from build123d import *

# Parameters (mm, degrees)
F0_R     = 4
F1_DEPTH = 2
F2_DEPTH = 5.5
F3_START = 5.5
F3_DEPTH = 1
F4_SIZE  = 0.99999


# Not quite as in the source:
# - a fillet or chamfer is up to 0.001 mm smaller than in the source, because OpenCascade refuses the exact size


with BuildPart() as f1:
    # F0 (on Front) → F1 (new body)
    with BuildSketch(Plane.XZ):
        Circle(F0_R)
        with BuildLine():
            ThreePointArc((-3.1622776602, 0.75), (0, 3.25), (3.1622776602, 0.75))
            Line((3.1622776602, 0.75), (3.5, 0.75))
            Line((3.5, 0.75), (3.5, -0.75))
            Line((3.5, -0.75), (3.1622776602, -0.75))
            ThreePointArc((3.1622776602, -0.75), (0, -3.25), (-3.1622776602, -0.75))
            Line((-3.1622776602, -0.75), (-3.5, -0.75))
            Line((-3.5, -0.75), (-3.5, 0.75))
            Line((-3.5, 0.75), (-3.1622776602, 0.75))
        make_face(mode=Mode.SUBTRACT)
        with BuildLine():
            ThreePointArc((2.3848480035, -0.75), (2.4710443145, -0.3793942482), (2.5, 0))
            ThreePointArc((2.5, 0), (2.4710443145, 0.3793942482), (2.3848480035, 0.75))
            Line((2.3848480035, 0.75), (-2.3848480035, 0.75))
            ThreePointArc((-2.3848480035, 0.75), (-2.5, 0), (-2.3848480035, -0.75))
            Line((-2.3848480035, -0.75), (2.3848480035, -0.75))
        make_face()
        with BuildLine():
            ThreePointArc((-2.3848480035, -0.75), (0, -2.5), (2.3848480035, -0.75))
            Line((2.3848480035, -0.75), (-2.3848480035, -0.75))
        make_face()
        with BuildLine():
            Line((-2.3848480035, 0.75), (2.3848480035, 0.75))
            ThreePointArc((2.3848480035, 0.75), (0, 2.5), (-2.3848480035, 0.75))
        make_face()
        with BuildLine():
            Line((3.1622776602, -0.75), (2.3848480035, -0.75))
            ThreePointArc((2.3848480035, -0.75), (0, -2.5), (-2.3848480035, -0.75))
            Line((-2.3848480035, -0.75), (-3.1622776602, -0.75))
            ThreePointArc((-3.1622776602, -0.75), (0, -3.25), (3.1622776602, -0.75))
        make_face()
        with BuildLine():
            ThreePointArc((-2.3848480035, 0.75), (0, 2.5), (2.3848480035, 0.75))
            Line((2.3848480035, 0.75), (3.1622776602, 0.75))
            ThreePointArc((3.1622776602, 0.75), (0, 3.25), (-3.1622776602, 0.75))
            Line((-3.1622776602, 0.75), (-2.3848480035, 0.75))
        make_face()
        with BuildLine():
            ThreePointArc((-2.3848480035, -0.75), (-2.5, 0), (-2.3848480035, 0.75))
            Line((-2.3848480035, 0.75), (-3.1622776602, 0.75))
            ThreePointArc((-3.1622776602, 0.75), (-3.25, 0), (-3.1622776602, -0.75))
            Line((-3.1622776602, -0.75), (-2.3848480035, -0.75))
        make_face()
        with BuildLine():
            ThreePointArc((2.3848480035, 0.75), (2.4710443145, 0.3793942482), (2.5, 0))
            ThreePointArc((2.5, 0), (2.4710443145, -0.3793942482), (2.3848480035, -0.75))
            Line((2.3848480035, -0.75), (3.1622776602, -0.75))
            ThreePointArc((3.1622776602, -0.75), (3.2279949191, -0.3775563564), (3.25, 0))
            ThreePointArc((3.25, 0), (3.2279949191, 0.3775563564), (3.1622776602, 0.75))
            Line((3.1622776602, 0.75), (2.3848480035, 0.75))
        make_face()
        with BuildLine():
            Line((3.5, 0.75), (3.1622776602, 0.75))
            ThreePointArc((3.1622776602, 0.75), (3.2279949191, 0.3775563564), (3.25, 0))
            ThreePointArc((3.25, 0), (3.2279949191, -0.3775563564), (3.1622776602, -0.75))
            Line((3.1622776602, -0.75), (3.5, -0.75))
            Line((3.5, -0.75), (3.5, 0.75))
        make_face()
        with BuildLine():
            ThreePointArc((-3.1622776602, -0.75), (-3.25, 0), (-3.1622776602, 0.75))
            Line((-3.1622776602, 0.75), (-3.5, 0.75))
            Line((-3.5, 0.75), (-3.5, -0.75))
            Line((-3.5, -0.75), (-3.1622776602, -0.75))
        make_face()
    extrude(amount=F1_DEPTH)

    # F0 (on Front) → F2 (join)
    with BuildSketch(Plane.XZ):
        with BuildLine():
            Line((-2.3848480035, 0.75), (2.3848480035, 0.75))
            ThreePointArc((2.3848480035, 0.75), (0, 2.5), (-2.3848480035, 0.75))
        make_face()
        with BuildLine():
            ThreePointArc((-2.3848480035, -0.75), (0, -2.5), (2.3848480035, -0.75))
            Line((2.3848480035, -0.75), (-2.3848480035, -0.75))
        make_face()
    extrude(amount=F2_DEPTH)

    # F0 (on Front) → F3 (join)
    with BuildSketch(Plane.XZ.offset(F3_START)):
        with BuildLine():
            Line((3.1622776602, -0.75), (2.3848480035, -0.75))
            ThreePointArc((2.3848480035, -0.75), (0, -2.5), (-2.3848480035, -0.75))
            Line((-2.3848480035, -0.75), (-3.1622776602, -0.75))
            ThreePointArc((-3.1622776602, -0.75), (0, -3.25), (3.1622776602, -0.75))
        make_face()
        with BuildLine():
            ThreePointArc((-2.3848480035, 0.75), (0, 2.5), (2.3848480035, 0.75))
            Line((2.3848480035, 0.75), (3.1622776602, 0.75))
            ThreePointArc((3.1622776602, 0.75), (0, 3.25), (-3.1622776602, 0.75))
            Line((-3.1622776602, 0.75), (-2.3848480035, 0.75))
        make_face()
        with BuildLine():
            Line((-2.3848480035, 0.75), (2.3848480035, 0.75))
            ThreePointArc((2.3848480035, 0.75), (0, 2.5), (-2.3848480035, 0.75))
        make_face()
        with BuildLine():
            ThreePointArc((-2.3848480035, -0.75), (0, -2.5), (2.3848480035, -0.75))
            Line((2.3848480035, -0.75), (-2.3848480035, -0.75))
        make_face()
    extrude(amount=F3_DEPTH)

    # F4 (size 1 in the source; OpenCascade refuses exactly that, so slightly less here)
    f4_edges = [f1.edges().sort_by_distance(p)[0] for p in [
        (0, -6.5, 3.25),
        (0, -6.5, -3.25),
    ]]
    chamfer(f4_edges, length=F4_SIZE)


solid = f1.part
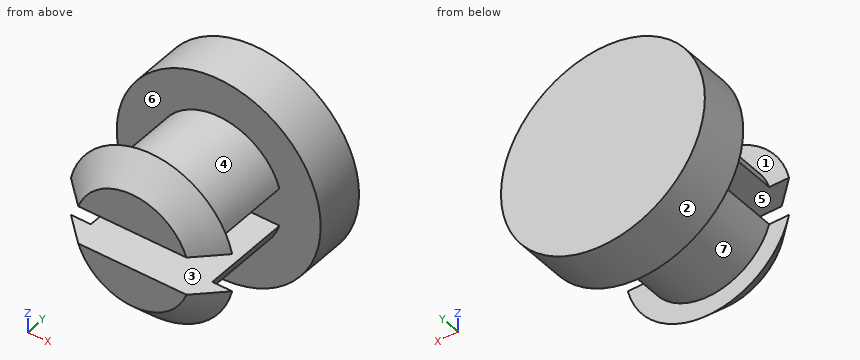
Could you check a few things on this model? Use its own coordinates, in mm. Face numbers are marked on the shaded views. A direction names the side the tool comes from. Give positions to 0.01 mm unless a question says otherwise; leave off trailing zeros. Order: outer loops, then holes, each group sorted by start corner. A loop starts at its lowest first (then second) coordinate and runs counter-clockwise, first axis right, second up. Notation, with made-up numbers: (-21.5, 46) - (15.5, 46) arc R23 cw to (15.5, 85) - close; hole circle Ø1 at (-34, -33). An arc over 180 degrees is marked (long way). One line per question, with ' | ' between items. Start each with the question number.
Item 1: I want a section at B-B on z = 0. Write out the boundary of the cut face in (x, y).
Item 2: I'm going to push flat-ended pins straight in: pin 1 Ø1 at (y, z) = (-1.5, 0.5) entering from -X; pin 2 Ø2 at (x, y) = (0.5, -4) entering from -Z; pin 3 Ø3.5 at (x, y) = (1.5, -3.5) entering from +Z. Where does each tip first touch, or does it pass through?
Item 3: I want a section at D-D on x = 3. Give the number of separate pieces and of enclosed holes in the cut face, then the cut area to 3 significant figures.
Item 4: I want a section at C-C on y = -1. Write out the boundary of the cut face in (x, z), then the cut area to 3 significant figures.
Item 5: I need wall thicknesses on probe 1 along Y at (x, z) = (2.5, 2.25); probe 2 along Z at (x, y) = (-1, -4.75); probe 3 along Z at (x, y) = (0.5, -4.5). Which ranges of each line are inside material? Lowest first, please. Write a range as [from, to].
Item 6: Thinking about a two-plate mould opening in Z: for the marked faces 1, 2 and 3, which applies, pulls with the +Z half, pulls with the -Z half, needs draft (parallel to the pull), parting line crosses it, or undercut?
Item 7: For the marked faces 4, 5, 6 and 7, which set-ups out of +Z, -Z, +X, -X, +Y, -Y let a thin tool reach every point of the face, with its end or its side?
Verdict:
1) outline: (-4, -2) - (4, -2) - (4, 0) - (-4, 0) - close
2) pin 1: x = -4 | pin 2: z = -2.5 | pin 3: z = 3.95
3) separate pieces: 3 | enclosed holes: 0 | area: 10.7 mm^2
4) outline: circle Ø8 at (0, 0) | area: 50.3 mm^2
5) probe 1: [-2, 0] | probe 2: [-2.29, -0.75], [0.75, 2.29] | probe 3: [-2.45, -0.75], [0.75, 2.45]
6) face 1: needs draft | face 2: parting line crosses it | face 3: undercut
7) face 4: +Z | face 5: +X, -X, -Y | face 6: none | face 7: -Z
